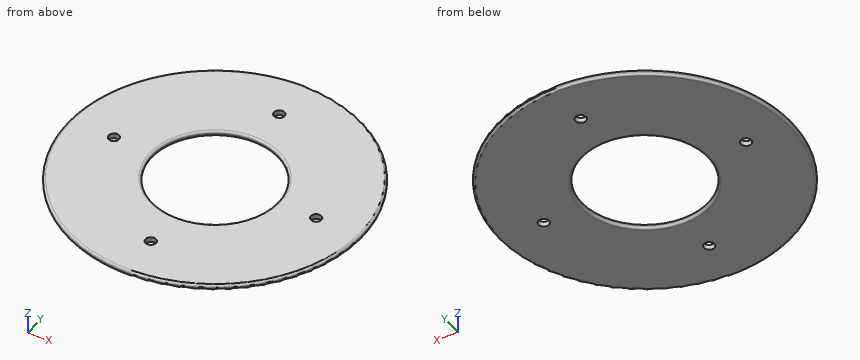
from build123d import *

# Parameters (mm, degrees)
SKETCH1_R           = 88.9
BOSS_EXTRUDE1_DEPTH = 3.175
FILLET1_R           = 1.27
SKETCH2_R           = 38.1
SKETCH2_R_2         = 3.175
CUT_EXTRUDE1_DEPTH  = 12.7
FILLET2_R           = 1.27


with BuildPart() as part:
    # Sketch1 → Boss-Extrude1 (new body)
    with BuildSketch(Plane.XY):
        Circle(SKETCH1_R)
    extrude(amount=BOSS_EXTRUDE1_DEPTH)

    # Fillet1
    fillet1_edges = [part.edges().sort_by_distance(p)[0] for p in [
        (-88.9, 0, 0),
        (-88.9, 0, 3.175),
    ]]
    fillet(fillet1_edges, radius=FILLET1_R)

    # Sketch2 → Cut-Extrude1 (cut)
    with BuildSketch(Plane.XY.offset(3.175)):
        Circle(SKETCH2_R)
        with Locations((0, 61.9125)):
            Circle(SKETCH2_R_2)
        with Locations((61.9125, 0)):
            Circle(SKETCH2_R_2)
        with Locations((0, -61.9125)):
            Circle(SKETCH2_R_2)
        with Locations((-61.9125, 0)):
            Circle(SKETCH2_R_2)
    extrude(amount=-CUT_EXTRUDE1_DEPTH, mode=Mode.SUBTRACT)

    # Fillet2
    fillet2_edges = [part.edges().sort_by_distance(p)[0] for p in [
        (-38.1, 0, 0),
        (-38.1, 0, 3.175),
    ]]
    fillet(fillet2_edges, radius=FILLET2_R)


solid = part.part
Can you work these out from the model? Positions are in its coordinate system, mm. Coordinates: 2 decimals unless noted, no trailing zeros. Loops run counter-clockwise (first coordinate to the right, second up) from the corner with the lowest first, then second, coordinate; pieces in that order, holes last. Notation, with made-up numbers: M 36.25,72 L 44.25,72 A13 ccw 44.25,96 Z; hole C -14,89 d6. An arc over 180 degrees is marked long. Return JSON: item names as keys, results as strings. Group by question number.
Item 1: If I drill on L1, parallel to Y at x = 0, z = 1.85; L2, parallel to Y at x = 0, z = 2.3; L3, parallel to X at y = 59, z = 2.95, over which ranges is the centre line in solid material (lowest first)? Write a range as from..to.
Item 2: I'm going to push flat-ended pins straight in: pin 1 Ø5 at (x, y) = (-61.91, 0) entering from +Z; pin 2 Ø1 at (x, z) = (33.5, 0.5) entering from -Y; pin 3 Ø10 at (x, y) = (61.91, 0) entering from -Z. Where does each tip first touch, or does it pass through?
Item 3: Imagine slicing it at C-C (z = 0.6). Give the number of separate pieces and of enclosed holes in the cut face, and give its area (3 significant figures).
Item 4: Imagine slicing it at A-A (y = 0). Please give me the cut outline in (x, z) (1 decimal).
Verdict:
{
 "1": {"L1": "y = -88.9..-65.09, -58.74..-38.1, 38.1..58.74, 65.09..88.9", "L2": "y = -88.84..-65.09, -58.74..-38.16, 38.16..58.74, 65.09..88.84", "L3": "x = -65.76..-1.26, 1.26..65.76"},
 "2": {"pin 1": "passes through", "pin 2": "stops at y = -82.41", "pin 3": "stops at z = 0"},
 "3": {"separate pieces": "1", "enclosed holes": "5", "area": "20,000 mm^2"},
 "4": {"outline": "M -88.9,1.3 A1.3 ccw -87.6,0 L -65.1,0 L -65.1,3.2 L -87.6,3.2 A1.3 ccw -88.9,1.9 Z; M -58.7,0 L -39.4,0 A1.3 ccw -38.1,1.3 L -38.1,1.9 A1.3 ccw -39.4,3.2 L -58.7,3.2 Z; M 38.1,1.3 A1.3 ccw 39.4,0 L 58.7,0 L 58.7,3.2 L 39.4,3.2 A1.3 ccw 38.1,1.9 Z; M 65.1,0 L 87.6,0 A1.3 ccw 88.9,1.3 L 88.9,1.9 A1.3 ccw 87.6,3.2 L 65.1,3.2 Z"}
}
